from build123d import *

# Parameters (mm, degrees)
F0_W     = 100
F0_H     = 88
F1_DEPTH = 12
F2_R     = 3
F3_DEPTH = 11.5
F4_R     = 3
F5_DEPTH = 12.001


with BuildPart() as f1:
    # F0 (on Front) → F1 (new body)
    with BuildSketch(Plane.XZ):
        with Locations((50, 44)):
            Rectangle(F0_W, F0_H)
    extrude(amount=F1_DEPTH)

    # F2 (on face) → F3 (join)
    with BuildSketch(Plane(origin=(0, 0, 0), x_dir=(1, 0, 0), z_dir=(0, 0, -1))):
        with Locations((7.5, 6)):
            Circle(F2_R)
        with Locations((92.5, 6)):
            Circle(F2_R)
    extrude(amount=F3_DEPTH)

    # F4 (on face) → F5 (cut, through all)
    with BuildSketch(Plane.XZ.offset(12)):
        with Locations((50, 68)):
            Circle(F4_R)
    extrude(amount=-F5_DEPTH, mode=Mode.SUBTRACT)


solid = f1.part
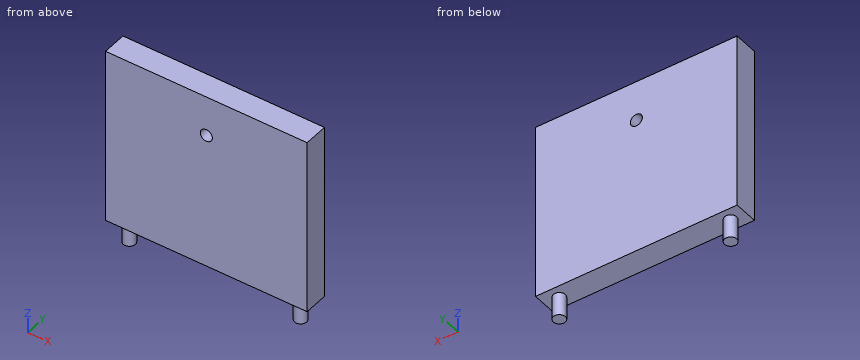
Verification items for the finished model (mm, model axes). Round coordinates to 2 decimals unless told otherwise and drop trailing zeros. Write each loop counter-clockwise with the first axis right and the second up, starting at its lowest first coordinate (ties: lowest second). Pieces come first, ordered by that corner, then holes.
(1) Section check A-A (z = 68). Enter the section's corners in (x, y).
Returned:
outline: (0, -12) - (47, -12) - (47, 0) - (0, 0) - close; (53, -12) - (100, -12) - (100, 0) - (53, 0) - close
(2) Section check B-B (y = -6). Enter the section's corners in (x, z), plus the area to 3 significant figures.
Returned:
outline: (0, 0) - (4.5, 0) - (4.5, -11.5) - (10.5, -11.5) - (10.5, 0) - (89.5, 0) - (89.5, -11.5) - (95.5, -11.5) - (95.5, 0) - (100, 0) - (100, 88) - (0, 88) - close; hole circle Ø6 at (50, 68)
area: 8,910 mm2
(3) Material ranges on line 1 (Z direction, x = 50, y = -7.5); line 2 (Z direction, x = 91.5, y = -2); line 3 (X direction, y = -7.75, z = 65.5), recorded low to high.
Returned:
line 1: z = 0 to 65, 71 to 88
line 2: z = 0 to 88
line 3: x = 0 to 48.34, 51.66 to 100
(4) Section check C-C (x = 7.5). Enter the section's corners in (y, z), plus the area to 4 significant figures.
Returned:
outline: (-12, 0) - (-9, 0) - (-9, -11.5) - (-3, -11.5) - (-3, 0) - (0, 0) - (0, 88) - (-12, 88) - close
area: 1,125 mm2
(5) Depth check by flat-ended pin: pin 1 Ø3 at (y, z) = (-4, 21) entering from -X; pin 2 Ø5.5 at (x, z) = (50, 68) entering from -Y. Enter the tip coordinate at first touch or a pass-through.
Returned:
pin 1: stops at x = 0
pin 2: passes through
(6) Section check D-D (x = 48.5). Enter the section's corners in (y, z).
Returned:
outline: (-12, 0) - (0, 0) - (0, 65.4) - (-12, 65.4) - close; (-12, 70.6) - (0, 70.6) - (0, 88) - (-12, 88) - close
